Read the model definition and answer for the solid it produces. Units are mm, in the model's axes. A direction names the side the tool comes from. Coordinates: 2 decimals unless noted, no trailing zeros. Loops run counter-clockwise (first coordinate to the right, second up) from the corner with the lowest first, then second, coordinate; pieces in that order, holes last.
Q1. Section A-A (x = 0) is taken. Give the vertices of the cut face in (y, z).
Q2. Section D-D (y = 1) is taken. Count the separate pieces of the cut face and the enclosed holes in it, then the cut area to 3 significant figures.
Q3. Section C-C (z = -12.25) is taken. Give the vertices of the cut face in (x, y).
Q4. Which of the six approach directions +Z, -Z, +X, -X, +Y, -Y give full straight-line access (tool end or side, diameter ignored) to faces 1 (the face through (-0.89, 16.14, 0.85)), 2 (the face through (-13, -1, 1.732)), 3 (the face through (-9.139, -14.334, -7.156))?
Q5. Straight lines are drawn through the part: line 1 (X direction, y = 0, z = -11); line 2 (Y direction, x = 0, z = 0.6); line 3 (Z direction, x = -13, y = 5.5). For each, find the intervals that lie inside material, in ascending order.
Q6. Section B-B (z = 2.5) is taken. Give the vertices of the cut face in (x, y), then the cut area to 3 significant figures.
Q7. Flat-ended cylindrical pins translate along their axes: P1, Ø5.5, axis at x = 14.75, y = 0, coming from the -Z side; P2, Ø4, axis at x = -14.75, y = 0, coming from the -Z side; P3, Ø2, axis at x = -4, y = 4.5, coming from the -Z side; P4, Ø5, axis at x = -14.75, y = 0, coming from the +Z side. Find the tip coordinate at first contact, or state that the pin passes through.
from build123d import *

# Parameters (mm, degrees)
F3_D           = 3.3
F3_DEPTH       = 8
F3_START       = 0.2679493
F3_CBORE_D     = 6.5
F3_CBORE_DEPTH = 3
F3_TIP         = 0.9914200214


with BuildPart() as f1:
    # F0 (on Front) → F1 (revolve)
    with BuildSketch(Plane.XZ):
        with BuildLine():
            Line((-16.5, 0), (0, 0))
            Line((0, 0), (0, 5))
            Line((0, 5), (-17, 5))
            ThreePointArc((-17, 5), (-18.4142135624, 4.4142135624), (-19, 3))
            Line((-19, 3), (-19, -13.5))
            ThreePointArc((-19, -13.5), (-18.8535533906, -13.8535533906), (-18.5, -14))
            Line((-18.5, -14), (-17, -14))
            Line((-17, -14), (-17, -0.5))
            ThreePointArc((-17, -0.5), (-16.8535533906, -0.1464466094), (-16.5, 0))
        make_face()
    revolve(axis=Axis((0, 0, 2.5), (0, 0, 1)))

    # F3
    # its depths count from where the whole tool has entered the part; down to there all is cleared
    with Locations(Plane.XY.offset(5).offset(-F3_START)):
        with Locations((0, 14.75), (14.75, 0), (0, -14.75), (-14.75, 0)):
            CounterBoreHole(F3_D / 2, F3_CBORE_D / 2, F3_CBORE_DEPTH, depth=F3_DEPTH)
            with Locations((0, 0, -(F3_DEPTH + F3_TIP / 2))):  # 118° drill point
                Cone(0, F3_D / 2, F3_TIP, mode=Mode.SUBTRACT)


solid = f1.part
Numbers:
1. outline: (-19, -13.5) arc R0.5 ccw to (-18.5, -14) - (-17, -14) - (-17, -0.5) arc R0.5 cw to (-16.5, 0) - (-16.4, 0) - (-16.4, 1.73) - (-18, 1.73) - (-18, 4.73) arc R2 ccw to (-19, 3) - close; (-13.1, 0) - (13.1, 0) - (13.1, 1.73) - (11.5, 1.73) - (11.5, 5) - (-11.5, 5) - (-11.5, 1.73) - (-13.1, 1.73) - close; (16.4, 0) - (16.5, 0) arc R0.5 cw to (17, -0.5) - (17, -14) - (18.5, -14) arc R0.5 ccw to (19, -13.5) - (19, 3) arc R2 ccw to (18, 4.73) - (18, 1.73) - (16.4, 1.73) - close
2. separate pieces: 3
2. enclosed holes: 0
2. area: 195 mm2
3. outline: circle Ø38 at (0, 0); hole circle Ø34 at (0, 0)
4. face 1: +Z, -Z
4. face 2: +Z
4. face 3: -Z
5. line 1: x = -19 to -17, 17 to 19
5. line 2: y = -19 to -16.4, -13.1 to 13.1, 16.4 to 19
5. line 3: z = 0 to 5
6. outline: circle Ø38 at (0, 0); hole circle Ø6.5 at (-14.75, 0); hole circle Ø6.5 at (0, -14.75); hole circle Ø6.5 at (0, 14.75); hole circle Ø6.5 at (14.75, 0)
6. area: 1,000 mm2
7. P1: stops at z = -14
7. P2: stops at z = -0.07
7. P3: stops at z = 0
7. P4: stops at z = 1.73
